Could you check a few things on this drawing? It's one solid part, dimensions in mm from its lowest x, y, z. Coordinates: 2 decimals unless noted, no trailing zeros. Order: outer loops, then holes, each group sorted by start corner. A loop starts at its lowest first (then second) coordinate and runs counter-clockwise, first axis right, second up.
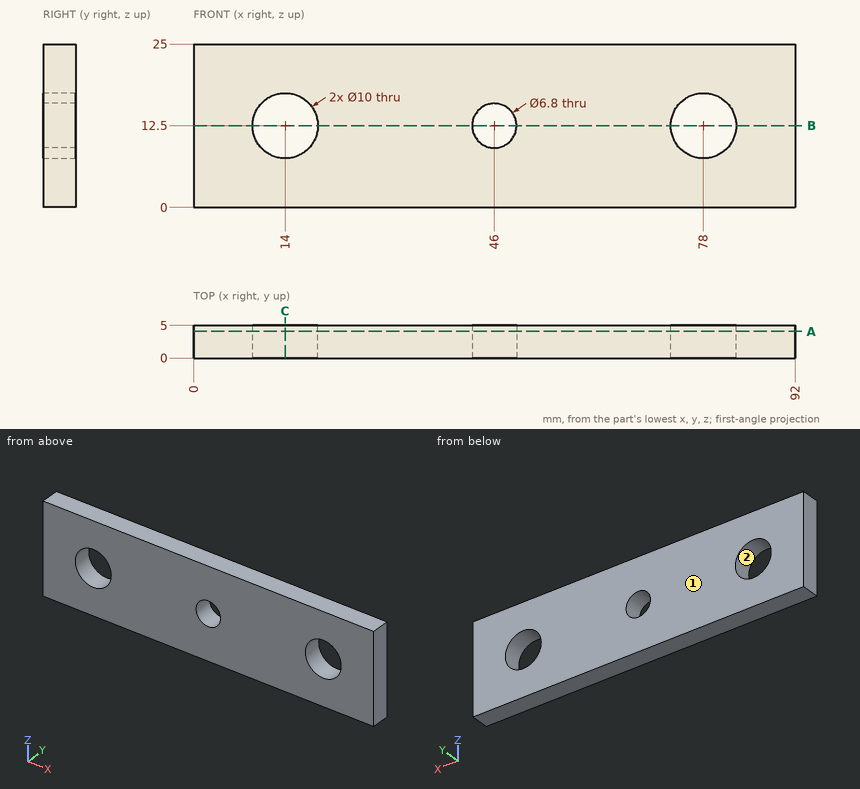
Item 1: Suppose I cut it at C-C (x = 14). List the corners of the cut face in (y, z) for me.
Item 2: Suppose I cut it at A-A (y = 4.1). List the corners of the cut face in (x, z) for me.
Item 3: Thinking about a two-plate mould opening in Z: for the marked faces 1 and 2, which applies, +Z half, -Z half, draft (parallel to the pull), parting line (faces both ways), or undercut?
Item 4: Suppose I cut it at B-B (z = 12.5). List the corners of the cut face in (x, y) for me, and give its area (3 significant figures).
Item 5: I need wall thicknesses on line 1 (X direction, y = 1.15, z = 12.5); line 2 (X direction, y = 1.75, z = 16); line 3 (Z direction, x = 48, y = 3.8). Which ranges of each line are inside material? Lowest first, please.
Geometry results:
1. outline: (0, 0) - (5, 0) - (5, 7.5) - (0, 7.5) - close; (0, 17.5) - (5, 17.5) - (5, 25) - (0, 25) - close
2. outline: (0, 0) - (92, 0) - (92, 25) - (0, 25) - close; hole circle Ø10 at (14, 12.5); hole circle Ø6.8 at (46, 12.5); hole circle Ø10 at (78, 12.5)
3. face 1: draft
3. face 2: undercut
4. outline: (0, 0) - (9, 0) - (9, 5) - (0, 5) - close; (19, 0) - (42.6, 0) - (42.6, 5) - (19, 5) - close; (49.4, 0) - (73, 0) - (73, 5) - (49.4, 5) - close; (83, 0) - (92, 0) - (92, 5) - (83, 5) - close
4. area: 326 mm2
5. line 1: x = 0 to 9, 19 to 42.6, 49.4 to 73, 83 to 92
5. line 2: x = 0 to 10.43, 17.57 to 74.43, 81.57 to 92
5. line 3: z = 0 to 9.75, 15.25 to 25
